Autodesk Inventor part; units mm, degrees
ref_plane "YZ Plane" through (0, 0, 0) normal (1, 0, 0) x (0, 1, 0)
ref_plane "XZ Plane" through (0, 0, 0) normal (0, 1, 0) x (-1, 0, 0)
ref_plane "XY Plane" through (0, 0, 0) normal (0, 0, 1) x (1, 0, 0)
sketch "スケッチ1" plane through (0, 0, 0) normal (0, 0, 1) x (1, 0, 0)
  arc A0 (-16.2703, -9.5731) -> (-13.6889, -8.0827) centre (-16.2703, -6.5923) ccw
  arc A1 (-16.2703, -9.5731) -> (-17.2313, -10.1279) centre (-16.2703, -10.6827) ccw
  arc A2 (-17.2313, -10.1279) -> (-17.2313, -11.2375) centre (-16.2703, -10.6827) ccw
  arc A3 (-17.2313, -14.2183) -> (-17.2313, -11.2375) centre (-19.8127, -12.7279) ccw
  arc A4 (-17.2313, -14.2183) -> (-17.2313, -15.3279) centre (-16.2703, -14.7731) ccw
  arc A5 (-17.2313, -15.3279) -> (-16.2703, -15.8827) centre (-16.2703, -14.7731) ccw
  arc A6 (-13.6889, -17.3731) -> (-16.2703, -15.8827) centre (-16.2703, -18.8635) ccw
  arc A7 (-13.6889, -17.3731) -> (-12.7279, -17.9279) centre (-12.7279, -16.8183) ccw
  arc A8 (-12.7279, -17.9279) -> (-11.767, -17.3731) centre (-12.7279, -16.8183) ccw
  arc A9 (-9.1855, -15.8827) -> (-11.767, -17.3731) centre (-9.1855, -18.8635) ccw
  arc A10 (-9.1855, -15.8827) -> (-8.2246, -15.3279) centre (-9.1855, -14.7731) ccw
  arc A11 (-8.2246, -15.3279) -> (-8.2246, -14.2183) centre (-9.1855, -14.7731) ccw
  arc A12 (-8.2246, -11.2375) -> (-8.2246, -14.2183) centre (-5.6431, -12.7279) ccw
  arc A13 (-8.2246, -11.2375) -> (-8.2246, -10.1279) centre (-9.1855, -10.6827) ccw
  arc A14 (-8.2246, -10.1279) -> (-9.1855, -9.5731) centre (-9.1855, -10.6827) ccw
  arc A15 (-11.767, -8.0827) -> (-9.1855, -9.5731) centre (-9.1855, -6.5923) ccw
  arc A16 (-11.767, -8.0827) -> (-12.7279, -7.5279) centre (-12.7279, -8.6375) ccw
  arc A17 (-12.7279, -7.5279) -> (-13.6889, -8.0827) centre (-12.7279, -8.6375) ccw
  circle A18 centre (-12.7279, -12.7279) radius 1.5 construction
  circle A19 centre (-12.7279, -12.7279) radius 1.25
  circle A20 centre (-12.7279, -12.7279) radius 6
  point P0 (0, 0)
  point P1 (0, 0)
  dimension "d0" = 2.5
extrude "押し出し1" add sketch "スケッチ1" against normal blind 1 contours A0 A17 A16 A15 A14 A13 A12 A11 A10 A9 A8 A7 A6 A5 A4 A3 A2 A1 | A20
extrude "押し出し2" add sketch "スケッチ1" along normal blind 4 contours A0 A17 A16 A15 A14 A13 A12 A11 A10 A9 A8 A7 A6 A5 A4 A3 A2 A1
sketch "書き出し" plane through (0, 0, 4) normal (0, 0, 1) x (1, 0, 0)
  arc A0 (-13.6889, -17.3731) -> (-11.767, -17.3731) centre (-12.7279, -16.8183) ccw
  arc A1 (-9.1855, -15.8827) -> (-11.767, -17.3731) centre (-9.1855, -18.8635) ccw
  arc A2 (-9.1855, -15.8827) -> (-8.2246, -14.2183) centre (-9.1855, -14.7731) ccw
  arc A3 (-8.2246, -11.2375) -> (-8.2246, -14.2183) centre (-5.6431, -12.7279) ccw
  arc A4 (-8.2246, -11.2375) -> (-9.1855, -9.5731) centre (-9.1855, -10.6827) ccw
  arc A5 (-11.767, -8.0827) -> (-9.1855, -9.5731) centre (-9.1855, -6.5923) ccw
  arc A6 (-11.767, -8.0827) -> (-13.6889, -8.0827) centre (-12.7279, -8.6375) ccw
  arc A7 (-16.2703, -9.5731) -> (-13.6889, -8.0827) centre (-16.2703, -6.5923) ccw
  arc A8 (-16.2703, -9.5731) -> (-17.2313, -11.2375) centre (-16.2703, -10.6827) ccw
  arc A9 (-17.2313, -14.2183) -> (-17.2313, -11.2375) centre (-19.8127, -12.7279) ccw
  arc A10 (-17.2313, -14.2183) -> (-16.2703, -15.8827) centre (-16.2703, -14.7731) ccw
  arc A11 (-13.6889, -17.3731) -> (-16.2703, -15.8827) centre (-16.2703, -18.8635) ccw
  circle A12 centre (-12.7279, -12.7279) radius 1.25
  arc A13 (-13.6889, -17.3731) -> (-16.2703, -15.8827) centre (-16.2703, -18.8635) ccw
  arc A14 (-17.2313, -14.2183) -> (-16.2703, -15.8827) centre (-16.2703, -14.7731) ccw
  arc A15 (-17.2313, -14.2183) -> (-17.2313, -11.2375) centre (-19.8127, -12.7279) ccw
  arc A16 (-16.2703, -9.5731) -> (-17.2313, -11.2375) centre (-16.2703, -10.6827) ccw
  arc A17 (-16.2703, -9.5731) -> (-13.6889, -8.0827) centre (-16.2703, -6.5923) ccw
  arc A18 (-11.767, -8.0827) -> (-13.6889, -8.0827) centre (-12.7279, -8.6375) ccw
  arc A19 (-11.767, -8.0827) -> (-9.1855, -9.5731) centre (-9.1855, -6.5923) ccw
  arc A20 (-8.2246, -11.2375) -> (-9.1855, -9.5731) centre (-9.1855, -10.6827) ccw
  arc A21 (-8.2246, -11.2375) -> (-8.2246, -14.2183) centre (-5.6431, -12.7279) ccw
  arc A22 (-9.1855, -15.8827) -> (-8.2246, -14.2183) centre (-9.1855, -14.7731) ccw
  arc A23 (-9.1855, -15.8827) -> (-11.767, -17.3731) centre (-9.1855, -18.8635) ccw
  arc A24 (-13.6889, -17.3731) -> (-11.767, -17.3731) centre (-12.7279, -16.8183) ccw
  circle A25 centre (-12.7279, -12.7279) radius 6
  circle A26 centre (-12.7279, -12.7279) radius 7.5
  point P0 (0, 0)
  dimension "d5" = 1.5
properties part number "原動節接続部v2内-1" material "アルミニウム 2014-T4"
The model under review builds one solid part; all positions refer to its coordinate system, in mm. A direction names the side the tool comes from. Coordinates: 2 decimals unless noted, no trailing zeros. Order: outer loops, then holes, each group sorted by start corner. A loop starts at its lowest first (then second) coordinate and runs counter-clockwise, first axis right, second up. Notation, with made-up numbers: (8.25, 48.5) -> (12.25, 48.5) arc R28 ccw to (12.25, 86.5) -> close; hole circle Ø11 at (58.5, 32.25). An arc over 180 degrees is marked (long way). Answer in a Markdown table with one row per item. Add a question column.
Item 1: To check wall thickness, follow probe 1 along X at (y, z) = (-12.75, 2.75); probe 2 along Y at (x, z) = (-11.75, -0.15); probe 3 along X at (y, z) = (-12, 0.25). State the ranges of each line that lie inside material, in increasing order.
Item 2: We need section C-C on y = -10.5. Write out the cut boundary in (x, z), plus the area to 3 significant figures.
Item 3: We need section A-A on z = 2.75. Write out the cut boundary in (x, y), plus the area to 3 significant figures.
Item 4: We need section B-B on x = -13. Write out the cut boundary in (y, z).
Item 5: Machinability: for faces 1 (the cylindrical face through (-8.638, -9.718, 1.972)), 2 (the cylindrical face through (-16.832, -9.726, 1.972)), 3 (the cylindrical face through (-17.38, -10.69, 1.97)), which of the approach directions +Z, -Z, +X, -X, +Y, -Y give a long, thin tool a straight path to every point of the face, cutting with its end or side? Answer none if there is none.
Item 6: Mouldability with a two-part tool opening along Y and no side actions: class faces 4 (the cylindrical face through (-12.18, -7.673, 1.972)), 5 (the cylindrical face through (-8.624, -12.75, 1.972)), 6 (the cylindrical face through (-14.8, -16.27, 1.97)) as +Y half, -Y half, draft (parallel to the pull), parting line (faces both ways), or undercut.
Item 7: Clearance check with a flat-ended pin moving along its axis: pin 1 (2 mm diameter, centred on x = -11, z = 2.5, fed in from +Y). State where the tip first meets the part, or that it passes through.
Item 8: We need section D-D on y = -12. Write out the cut boundary in (x, z), plus the area to 3 significant figures.
Final values:
| question | item | result |
|---|---|---|
| 1 | probe 1 | x = -16.83 to -13.98, -11.48 to -8.62 |
| 1 | probe 2 | y = -18.65 to -13.51, -11.95 to -6.81 |
| 1 | probe 3 | x = -16.92 to -13.74, -11.71 to -8.53 |
| 2 | outline | (-18.3, -1) -> (-7.16, -1) -> (-7.16, 0) -> (-8.09, 0) -> (-8.09, 4) -> (-17.36, 4) -> (-17.36, 0) -> (-18.3, 0) -> close |
| 2 | area | 48.2 mm2 |
| 3 | outline | (-17.23, -15.33) arc R1.11 ccw to (-16.27, -15.88) arc R2.98 cw to (-13.69, -17.37) arc R1.11 ccw to (-12.73, -17.93) arc R1.11 ccw to (-11.77, -17.37) arc R2.98 cw to (-9.19, -15.88) arc R1.11 ccw to (-8.22, -15.33) arc R1.11 ccw to (-8.22, -14.22) arc R2.98 cw to (-8.22, -11.24) arc R1.11 ccw to (-8.22, -10.13) arc R1.11 ccw to (-9.19, -9.57) arc R2.98 cw to (-11.77, -8.08) arc R1.11 ccw to (-12.73, -7.53) arc R1.11 ccw to (-13.69, -8.08) arc R2.98 cw to (-16.27, -9.57) arc R1.11 ccw to (-17.23, -10.13) arc R1.11 ccw to (-17.23, -11.24) arc R2.98 cw to (-17.23, -14.22) arc R1.11 ccw to start; hole circle Ø2.5 at (-12.73, -12.73) |
| 3 | area | 61.9 mm2 |
| 4 | outline | (-18.72, -1) -> (-13.95, -1) -> (-13.95, 4) -> (-17.89, 4) -> (-17.89, 0) -> (-18.72, 0) -> close; (-11.51, -1) -> (-6.73, -1) -> (-6.73, 0) -> (-7.56, 0) -> (-7.56, 4) -> (-11.51, 4) -> close |
| 5 | face 1 | +Z, +X, +Y |
| 5 | face 2 | +Z, -X, +Y |
| 5 | face 3 | +Z, -X |
| 6 | face 4 | +Y half |
| 6 | face 5 | undercut |
| 6 | face 6 | -Y half |
| 7 | pin 1 | stops at y = -7.8 |
| 8 | outline | (-18.68, -1) -> (-13.74, -1) -> (-13.74, 4) -> (-16.92, 4) -> (-16.92, 0) -> (-18.68, 0) -> close; (-11.71, -1) -> (-6.77, -1) -> (-6.77, 0) -> (-8.53, 0) -> (-8.53, 4) -> (-11.71, 4) -> close |
| 8 | area | 35.3 mm2 |
